Answer from the drawing. Dimensions are ordinates in mm from the lowest x, y and z of the part. A direction names the side the tool comes from. Coordinates: 2 decimals unless noted, no trailing zeros. Order: outer loops, then holes, each group sorted by start corner. A loop starts at its lowest first (then second) coordinate and runs counter-clockwise, first axis right, second up. Notation, with made-up numbers: (-0.75, 12.5) - (40.25, 12.5) arc R31 ccw to (40.25, 49.5) - close; hole circle Ø4 at (68, 23). An arc over 180 degrees is marked (long way). Answer as a JSON object with one key per item and string values. Group by question number.
1) Section A-A (z = 7.5) is taken. Give the vertices of the cut face in (x, y).
2) Each of these flat-tipped pins is pushed along its axis until it touches: P1, Ø5, axis at x = 16.5, z = 18.5, coming from the +Y side; P2, Ø4, axis at y = 8, z = 22.5, coming from the -X side; P3, Ø10, axis at x = 18, z = 24, coming from the +Y side (1 decimal). Where does it stop, or does it pass through?
3) Section B-B (x = 10.16) is taken. Give the vertices of the cut face in (y, z).
4) The mould has two halves that part along Y. Classify the marked faces 1, 2, 3 and 4: released by +Y, released by -Y, zero draft, split by the parting line, or undercut.
5) A tool of negligible diameter and unlimited length cuts with its end or side. For the marked faces 5 and 6, from which of +Z, -Z, +X, -X, +Y, -Y can it reach the whole face along a straight path? Write none if from no direction.
6) Find the intervals of material crossed by line 1 along Y through (x, z) = (9.75, 22); line 2 along X through (y, z) = (9.25, 18.5) (1 decimal); line 3 along X through (y, z) = (6.5, 30) (1 decimal), in increasing order.
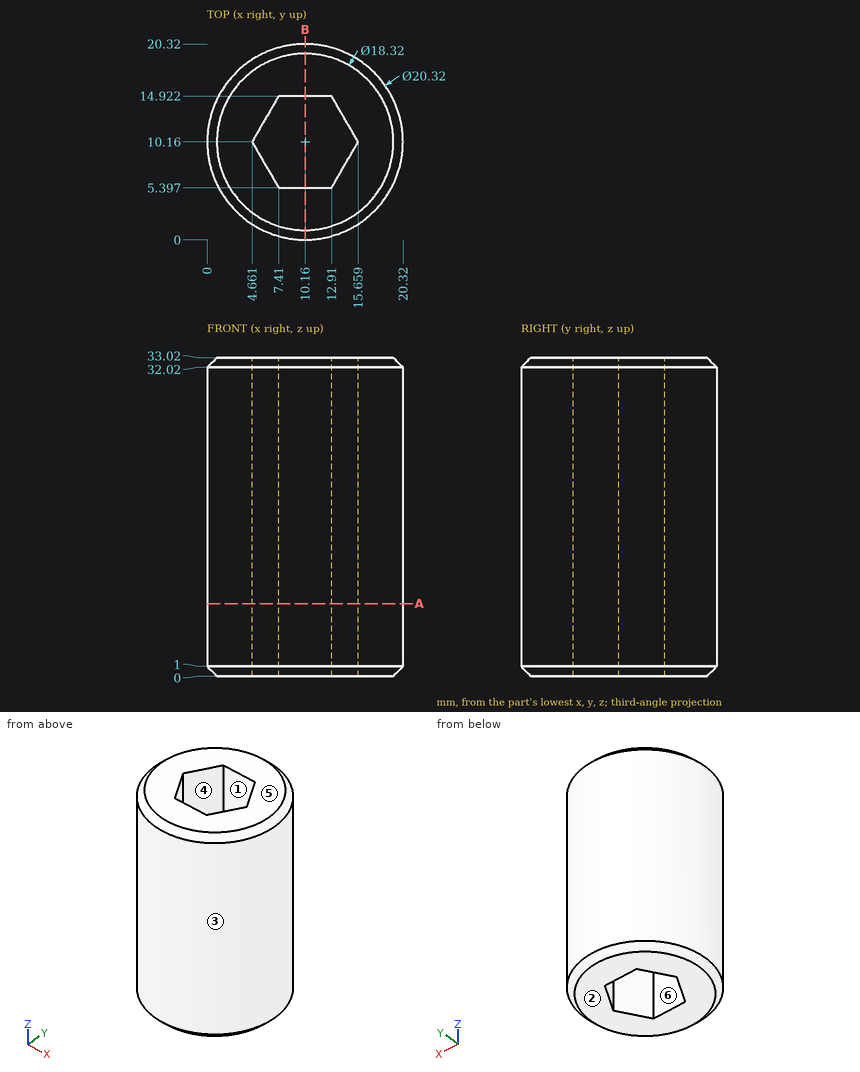
Report:
{
 "1": {"outline": "circle Ø20.32 at (10.16, 10.16); hole (4.66, 10.16) - (7.41, 5.4) - (12.91, 5.4) - (15.66, 10.16) - (12.91, 14.92) - (7.41, 14.92) - close"},
 "2": {"P1": "stops at y = 19.57", "P2": "stops at x = 0", "P3": "stops at y = 19.9"},
 "3": {"outline": "(0, 1) - (1, 0) - (5.4, 0) - (5.4, 33.02) - (1, 33.02) - (0, 32.02) - close; (14.92, 0) - (19.32, 0) - (20.32, 1) - (20.32, 32.02) - (19.32, 33.02) - (14.92, 33.02) - close"},
 "4": {"face 1": "undercut", "face 2": "zero draft", "face 3": "split by the parting line", "face 4": "undercut"},
 "5": {"face 5": "+Z, +X, -X, +Y, -Y", "face 6": "+Z, -Z"},
 "6": {"line 1": "y = 0.01 to 5.4, 14.92 to 20.31", "line 2": "x = 0 to 5.2, 15.1 to 20.3", "line 3": "x = 0.7 to 6.8, 13.5 to 19.6"}
}
